For this review, take the finished solid that the model builds, in its own axes (mm). Round coordinates to 2 decimals unless told otherwise and drop trailing zeros. Write each loop counter-clockwise with the first axis right and the second up, starting at its lowest first coordinate (ties: lowest second). Pieces come first, ordered by that corner, then holes. Notation, with made-up numbers: (48.5, 20) -> (82.5, 20) arc R20 ccw to (82.5, 49) -> close; hole circle Ø2 at (-32.5, -21.5). An arc over 180 degrees is marked (long way). Answer in a Markdown table with one row per item. Add a question column.
```python
from build123d import *

# Parameters (mm, degrees)
SKETCH1_R                 = 11.0998
SKETCH1_R_2               = 9.525
BOSS_EXTRUDE1_DEPTH       = 3.175
F_8_CLEARANCE_HOLE1_D     = 4.4958
F_8_CLEARANCE_HOLE1_DEPTH = 12.7
F_8_CLEARANCE_HOLE1_TIP   = 1.350674586
F_8_CLEARANCE_HOLE2_D     = 4.4958


with BuildPart() as part:
    # Sketch1 → Boss-Extrude1 (new body)
    with BuildSketch(Plane.XY):
        with BuildLine():
            Line((-188.264639147, 81.011774484), (56.809800323, 298.704514086))
            ThreePointArc((56.809800323, 298.704514086), (76.096805757, 305.388436009), (94.461024604, 296.476710194))
            Line((94.461024604, 296.476710194), (260.194034881, 109.897568099))
            ThreePointArc((260.194034881, 109.897568099), (271.059668812, 38.975929697), (210.82, 0))
            Line((210.82, 0), (-157.48, 0))
            ThreePointArc((-157.48, 0), (-200.811863601, 29.88880366), (-188.264639147, 81.011774484))
        make_face()
        with Locations((-157.48, 46.355)):
            Circle(SKETCH1_R, mode=Mode.SUBTRACT)
        with Locations((74.521510517, 278.765)):
            Circle(SKETCH1_R, mode=Mode.SUBTRACT)
        with Locations((210.82, 66.04)):
            Circle(SKETCH1_R, mode=Mode.SUBTRACT)
        with Locations((18.5166, 46.355)):
            Circle(SKETCH1_R_2, mode=Mode.SUBTRACT)
    extrude(amount=BOSS_EXTRUDE1_DEPTH)

    # #8 Clearance Hole1
    with Locations(Plane.XY.offset(3.175)):
        with Locations((36.477112242, 64.315512242), (36.477112242, 28.394487758), (0.556087758, 28.394487758), (0.556087758, 64.315512242)):
            Hole(F_8_CLEARANCE_HOLE1_D / 2, depth=F_8_CLEARANCE_HOLE1_DEPTH)
            with Locations((0, 0, -(F_8_CLEARANCE_HOLE1_DEPTH + F_8_CLEARANCE_HOLE1_TIP / 2))):  # 118° drill point
                Cone(0, F_8_CLEARANCE_HOLE1_D / 2, F_8_CLEARANCE_HOLE1_TIP, mode=Mode.SUBTRACT)

    # #8 Clearance Hole2 (through all)
    with Locations(Plane.XY.offset(3.175)):
        with Locations((17.768914495, 247.038768822), (36.758927911, 263.907064244), (110.26846103, 259.557542359), (127.136756453, 240.567528943), (208.528289616, 148.938453927), (225.396585039, 129.948440511), (270.394698688, 62.514995218), (253.027203769, 23.832796231), (172.72, 12.7), (147.32, 12.7), (-93.98, 12.7), (-119.38, 12.7), (-194.875991874, 32.144446994), (-151.345471312, 96.81921091), (-132.355457896, 113.687506333), (-68.58, 149.225), (-68.58, 92.075), (121.92, 92.075), (121.92, 149.225), (71.12, 200.025), (26.67, 120.65), (0.556087758, 75.2475), (56.436087758, 75.2475), (56.436087758, 17.4625), (0.556087758, 17.4625)):
            Hole(F_8_CLEARANCE_HOLE2_D / 2)


solid = part.part
```
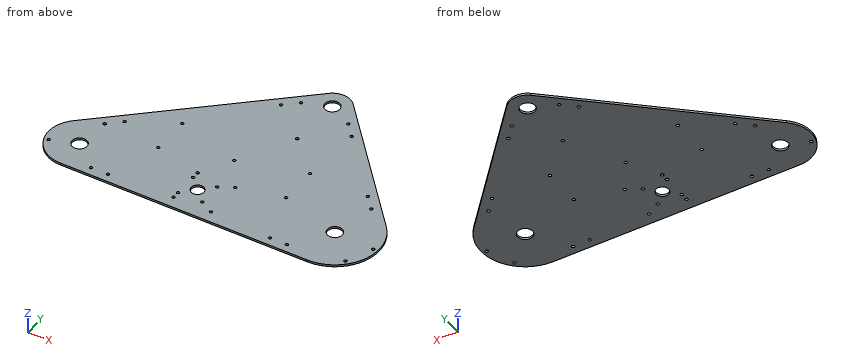
1. We need section A-A (z = 2.3). Count the separate pieces of the cut face and the enclosed holes in it, plus the area to 3 significant figures.
2. We need section B-B (x = -85.5). Write out the cut boundary in (y, z) (3 decimals).
3. Clearance check with flat-ended pins moving along their axes: pin 1 Ø2.5 at (x, y) = (56.44, 75.25) entering from -Z; pin 2 Ø1 at (x, z) = (-153, 1) entering from +Y; pin 3 Ø1.5 at (y, z) = (190, 1.5) entering from +X. State where each tip first meets the part, or that it passes through.
4. For L1, parallel to X at y = 92, z = 2.5; L2, parallel to Y at x = -157.5, z = 2.9; L3, parallel to Y at x = -93.5, z = 1.75, list the stretches that pass through material, from the lowest coordinate up. Write a range as [from, to].
Response:
| question | item | result |
|---|---|---|
| 1 | separate pieces | 1 |
| 1 | enclosed holes | 33 |
| 1 | area | 91,000 mm2 |
| 2 | outline | (0, 0) -> (172.295, 0) -> (172.295, 3.175) -> (0, 3.175) -> close |
| 3 | pin 1 | through |
| 3 | pin 2 | y = 112.78 |
| 3 | pin 3 | x = 189.71 |
| 4 | L1 | [-175.89, -70.83], [-66.33, 119.67], [124.17, 271.54] |
| 4 | L2 | [0, 35.26], [57.45, 108.34] |
| 4 | L3 | [0, 10.5], [14.9, 165.19] |
